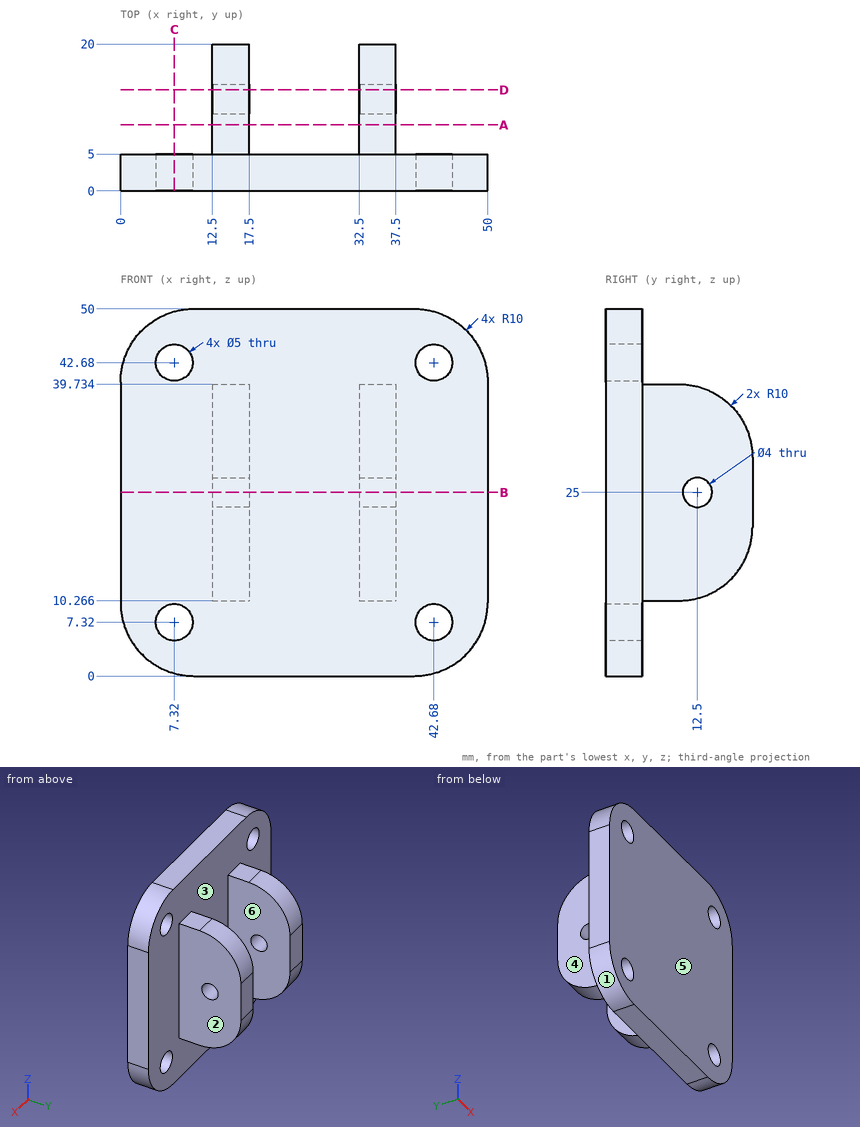
Design review of the part shown in the three views and the two pictorial views. Dimensions are in mm from the part's minimum x, y and z. A direction names the side the tool comes from. Give positions to 0.01 mm unless a question says otherwise; leave off trailing zeros. Loops run counter-clockwise (first coordinate to the right, second up) from the corner with the lowest first, then second, coordinate; pieces in that order, holes last. Notation, with made-up numbers: (-12.75, 31) -> (-0.75, 31) arc R24 cw to (-0.75, 48) -> close; hole circle Ø11 at (21.25, 42). An arc over 180 degrees is marked (long way). Write each question's results on one line, items separated by ' | '.
Q1. Wall thickness on L1, parallel to X at y = 14, z = 13.5; L2, parallel to X at y = 1.8, z = 42.68 (1 decimal); L3, parallel to Y at x = 47, z = 29.5: over which ranges is each line inside the solid? List them lowest first.
Reply:
L1: x = 12.5 to 17.5, 32.5 to 37.5 | L2: x = 0.4 to 4.8, 9.8 to 40.2, 45.2 to 49.6 | L3: y = 0 to 5
Q2. Take a section at C-C, the plane x = 7.32. Write out the cut boundary in (y, z).
Reply:
outline: (0, 0.37) -> (5, 0.37) -> (5, 4.82) -> (0, 4.82) -> close; (0, 9.82) -> (5, 9.82) -> (5, 40.18) -> (0, 40.18) -> close; (0, 45.18) -> (5, 45.18) -> (5, 49.63) -> (0, 49.63) -> close
Q3. Take a section at B-B, the plane z = 25. Write out the cut boundary in (x, y), plus the area to 3 significant figures.
Reply:
outline: (0, 0) -> (50, 0) -> (50, 5) -> (37.5, 5) -> (37.5, 10.5) -> (32.5, 10.5) -> (32.5, 5) -> (17.5, 5) -> (17.5, 10.5) -> (12.5, 10.5) -> (12.5, 5) -> (0, 5) -> close; (12.5, 14.5) -> (17.5, 14.5) -> (17.5, 20) -> (12.5, 20) -> close; (32.5, 14.5) -> (37.5, 14.5) -> (37.5, 20) -> (32.5, 20) -> close | area: 360 mm²
Q4. The part is to be moulded in two halves that separate along X. For the marked faces 3, 4, 5 and 6, say which applies: +X half, -X half, draft (parallel to the pull), parting line (faces both ways), or undercut.
Reply:
face 3: undercut | face 4: -X half | face 5: draft | face 6: undercut
Q5. Take a section at A-A, the plane y = 9. Write out the cut boundary in (x, z).
Reply:
outline: (12.5, 10.27) -> (17.5, 10.27) -> (17.5, 39.73) -> (12.5, 39.73) -> close; (32.5, 10.27) -> (37.5, 10.27) -> (37.5, 39.73) -> (32.5, 39.73) -> close
Q6. For pin 1 Ø6 at (x, z) = (15.5, 43) entering from +Y; pin 2 Ø4 at (x, y) = (15, 8) entering from +Z; pin 3 Ø4.5 at (x, z) = (7.32, 7.32) entering from +Y; pin 4 Ø10 at (x, y) = (12.5, 13.5) entering from -Z, all flat-tipped, find the tip position at first contact; note any pin that passes through.
Reply:
pin 1: stops at y = 5 | pin 2: stops at z = 39.73 | pin 3: passes through | pin 4: stops at z = 10.27
Q7. Take a section at D-D, the plane y = 13.75. Write out the cut boundary in (x, z) (1 decimal), plus the area to 3 significant figures.
Reply:
outline: (12.5, 11) -> (17.5, 11) -> (17.5, 23.4) -> (12.5, 23.4) -> close; (12.5, 26.6) -> (17.5, 26.6) -> (17.5, 39) -> (12.5, 39) -> close; (32.5, 11) -> (37.5, 11) -> (37.5, 23.4) -> (32.5, 23.4) -> close; (32.5, 26.6) -> (37.5, 26.6) -> (37.5, 39) -> (32.5, 39) -> close | area: 249 mm²
Q8. Machinability: for the marked faces 1 and 2, which of the approach directions +Z, -Z, +X, -X, +Y, -Y give a long, thin tool a straight path to every point of the face, cutting with its end or side? Answer none if there is none.
Reply:
face 1: -Z, -X, +Y, -Y | face 2: +Z, -Z, +X, +Y
